Autodesk Inventor part; units mm, degrees
ref_plane "YZ Plane" through (0, 0, 0) normal (1, 0, 0) x (0, 1, 0)
ref_plane "XZ Plane" through (0, 0, 0) normal (0, 1, 0) x (-1, 0, 0)
ref_plane "XY Plane" through (0, 0, 0) normal (0, 0, 1) x (1, 0, 0)
sketch "Sketch1" plane through (0, 0, 0) normal (0, 1, 0) x (-1, 0, 0)
  line L0 (0, 0) -> (60, 0)
  line L1 (60, 0) -> (60, -40)
  line L2 (60, -40) -> (0, -40)
  line L3 (0, -40) -> (0, 0)
  dimension "d0" = 60
  dimension "d1" = 40
extrude "Extrusion1" add sketch "Sketch1" along normal blind 35.4
sketch "Sketch2" plane through (0, 35.4, 0) normal (0, 1, 0) x (1, 0, 0)
  line L0 (-60, 0) -> (0, 0)
  line L1 (0, 40) -> (-60, 40)
  line L2 (-43.7, 6.3) -> (-43.7, 33.7)
  line L3 (-43.7, 33.7) -> (-16.3, 33.7)
  line L4 (-16.3, 33.7) -> (-16.3, 20)
  line L5 (-16.3, 20) -> (-16.3, 6.3)
  line L6 (-16.3, 6.3) -> (-43.7, 6.3)
  line L7 (-48.7, 38.7) -> (-48.7, 1.3)
  line L8 (-48.7, 1.3) -> (-11.3, 1.3)
  line L9 (-11.3, 1.3) -> (-11.3, 38.7)
  line L10 (-11.3, 38.7) -> (-48.7, 38.7)
  dimension "d9" = 5
extrude "Extrusion2" cut sketch "Sketch2" against normal blind 25.4 contours L2 L3 L4 L5 L6
sketch "Sketch3" plane through (-60, 0, 0) normal (0, 0, 1) x (1, 0, 0)
  line L0 (60, 0) -> (60, 35.4)
  line L1 (60, 35.4) -> (30, 35.4)
  line L2 (0, 35.4) -> (60, 35.4)
  line L3 (30, 35.4) -> (11.3, 35.4)
  line L4 (0, 0) -> (0, 35.4)
  line L5 (0, 0) -> (0, 10)
  line L6 (0, 10) -> (11.3, 35.4)
  line L7 (0, 35.4) -> (11.3, 35.4)
  line L8 (0, 35.4) -> (0, 10)
  line L9 (60, 0) -> (0, 0)
  line L10 (60, 35.4) -> (0, 35.4)
  line L11 (60, 0) -> (60, 35.4)
  line L12 (60, 10) -> (48.7, 35.4)
  line L13 (60, 35.4) -> (60, 10)
  dimension "d12" = 18.7
  dimension "d13" = 10
extrude "Extrusion3" cut sketch "Sketch3" against normal through all contours L12 L1 L0 | L4 L2 L6
sketch "Sketch4" plane through (0, 0, 0) normal (0, -1, 0) x (1, 0, 0)
  line L0 (-60, 0) -> (0, 0)
  line L1 (-11.3, -40) -> (-48.7, -40)
  circle A0 centre (-50, -10) radius 1.5
  circle A1 centre (-50, -30) radius 1.5
  circle A2 centre (-10, -30) radius 1.5
  circle A3 centre (-10, -10) radius 1.5
  dimension "d20" = 3
extrude "Extrusion4" cut sketch "Sketch4" against normal blind 10
properties part number "Tilt_Metal_Attachment"
Here's how the part is built. I have some questions about the finished solid (model axes, mm). A direction names the side the tool comes from. Give positions to 0.01 mm unless a question says otherwise; leave off trailing zeros. Write each loop counter-clockwise with the first axis right and the second up, starting at its lowest first coordinate (ties: lowest second). Pieces come first, ordered by that corner, then holes. Notation, with made-up numbers: (60, -39.75) -> (65, -39.75) arc R14 cw to (65, -13.75) -> close; hole circle Ø7 at (65, 41.25). An arc over 180 degrees is marked (long way). Use one line per item in the form item = value.
1) I'm going to push flat-ended pins straight in: pin 1 (1.5 mm diameter, centred on x = -10.5, z = -10, fed in from -Y); pin 2 (7.5 mm diameter, centred on y = 26.5, z = -13.5, fed in from -X); pin 3 (2.5 mm diameter, centred on x = -10, z = -30, fed in from +Y). Where does each tip first touch, or does it pass through?
Verdict:
pin_1 = 10
pin_2 = -54.33
pin_3 = 35.29
2) If I drill on L1, parallel to Z at x = -10, y = 6; L2, parallel to Z at x = -40, y = 16.5; L3, parallel to X at y = 15, z = -30, over which ranges is the centre line in solid material (lowest first)? Write a range as [from, to].
Verdict:
L1 = [-40, -31.5], [-28.5, -11.5], [-8.5, 0]
L2 = [-40, -33.7], [-6.3, 0]
L3 = [-57.78, -43.7], [-16.3, -2.22]
3) Suppose I cut it at D-D (z = -3.5). Please give me the cut outline in (x, y), and give its area (3 significant figures).
Verdict:
outline = (-60, 0) -> (0, 0) -> (0, 10) -> (-11.3, 35.4) -> (-48.7, 35.4) -> (-60, 10) -> close
area = 1,840 mm2
4) Suppose I cut it at C-C (x = -50). Please give me the cut outline in (y, z).
Verdict:
outline = (0, -40) -> (32.48, -40) -> (32.48, 0) -> (0, 0) -> (0, -8.5) -> (10, -8.5) -> (10, -11.5) -> (0, -11.5) -> (0, -28.5) -> (10, -28.5) -> (10, -31.5) -> (0, -31.5) -> close
5) We'd pull the mould along Z, two halves only. Please class faces 1 (the face through (-30, 0, -20)), 2 (the face through (-30, 17, -40)), 3 (the face through (-51.2, 4.9, -10.9)), 4 (the face through (-30, 17, 0)): +Z half, -Z half, draft (parallel to the pull), parting line (faces both ways), or undercut.
Verdict:
face_1 = draft
face_2 = -Z half
face_3 = undercut
face_4 = +Z half
6) Suppose I cut it at B-B (y = 20). Please give me the cut outline in (x, z).
Verdict:
outline = (-55.55, -40) -> (-4.45, -40) -> (-4.45, 0) -> (-55.55, 0) -> close; hole (-43.7, -33.7) -> (-16.3, -33.7) -> (-16.3, -6.3) -> (-43.7, -6.3) -> close
7) On a 3-axis mill with a long thin cutter (end or side, diameter ignored), from which of +Z, -Z, +X, -X, +Y, -Y can I reach the whole of each face in a straight line? I mean faces 5 (the face through (-43.7, 23, -20)), 6 (the face through (0, 5, -20)), 7 (the face through (-11.2, 4.9, -10.9)). Say none if no direction works.
Verdict:
face_5 = +Y
face_6 = +Z, -Z, +X, +Y, -Y
face_7 = -Y
8) Suppose I cut it at A-A (z = -30). Please give me the cut outline in (x, y).
Verdict:
outline = (-60, 0) -> (-51.5, 0) -> (-51.5, 10) -> (-48.5, 10) -> (-48.5, 0) -> (-11.5, 0) -> (-11.5, 10) -> (-8.5, 10) -> (-8.5, 0) -> (0, 0) -> (0, 10) -> (-11.3, 35.4) -> (-16.3, 35.4) -> (-16.3, 10) -> (-43.7, 10) -> (-43.7, 35.4) -> (-48.7, 35.4) -> (-60, 10) -> close
